Can you work these out from the model? Positions are in its coordinate system, mm. A direction names the side the tool comes from. Coordinates: 2 decimals unless noted, no trailing zeros. Order: outer loops, then holes, each group sorted by start corner. A loop starts at its lowest first (then second) coordinate and runs counter-clockwise, first axis right, second up. Notation, with made-up numbers: (17, -28.5) -> (43, -28.5) arc R22 cw to (43, 5.5) -> close; hole circle Ø9 at (26, 33.25). An arc over 180 degrees is marked (long way). Write item = value, one per line. Start each with the question number.
from build123d import *

# Parameters (mm, degrees)
SKETCH1_W               = 60
SKETCH1_H               = 60
BOSS_EXTRUDE1_DEPTH     = 85
SKETCH2_W               = 40
SKETCH2_H               = 35
CUT_EXTRUDE1_DEPTH      = 121.104121495
CUT_EXTRUDE2_DEPTH      = 99.488578018
CUT_EXTRUDE2_DEPTH_BACK = 99.488578018
SKETCH3_R               = 11


with BuildPart() as part:
    # Sketch1 → Boss-Extrude1 (new body)
    with BuildSketch(Plane(origin=(0, 0, 0), x_dir=(1, 0, 0), z_dir=(0, 1, 0))):
        with Locations((30, 30)):
            Rectangle(SKETCH1_W, SKETCH1_H)
    extrude(amount=BOSS_EXTRUDE1_DEPTH)

    # Sketch2 → Cut-Extrude1 (cut, through all)
    with BuildSketch(Plane(origin=(60, 0, 0), x_dir=(0, 0, -1), z_dir=(1, 0, 0))):
        with Locations((20, 52.5)):
            Rectangle(SKETCH2_W, SKETCH2_H)
    extrude(amount=-CUT_EXTRUDE1_DEPTH, mode=Mode.SUBTRACT)

    # Sketch3 → Cut-Extrude2 (cut, two sides: drawn at the far end of the back side and taken through both)
    with BuildSketch(Plane(origin=(0, 35, 0), x_dir=(1, 0, 0), z_dir=(0, 1, 0)).offset(-CUT_EXTRUDE2_DEPTH_BACK)):
        with Locations(Location((30, 20, 0), (0, 0, 270))):
            Circle(SKETCH3_R)
    extrude(amount=CUT_EXTRUDE2_DEPTH + CUT_EXTRUDE2_DEPTH_BACK, mode=Mode.SUBTRACT)


solid = part.part
(1) Imagine slicing it at B-B (z = -4.5). Write out the boundary of the cut face in (x, y), plus the area to 3 significant figures.
(2) If I drill on L1, parallel to Z at x = 30, y = 22; L2, parallel to Y at x = 30, z = -6; L3, parallel to X at y = 73, z = -20, over which ranges is the centre line in solid material (lowest first)? Write a range as from..to.
(3) Imagine slicing it at C-C (z = -20). Write out the boundary of the cut face in (x, y).
(4) For P1, Ø2, axis at x = 52.5, y = 41.5, coming from the +Z side, with a flat end and sliding along its axis, tell me the tip position at first contact or that it passes through.
(5) Imagine slicing it at D-D (x = 46.5). Write out the boundary of the cut face in (y, z), plus the area to 3 significant figures.
(6) For faces 1 (the face through (30, 77, 0)), 2 (the face through (37, 35, -11)), which set-ups out of +Z, -Z, +X, -X, +Y, -Y let a thin tool reach every point of the face, with its end or its side?
(7) Imagine slicing it at A-A (x = 30). Write out the boundary of the cut face in (y, z), plus the area to 3 significant figures.
(8) Thinking about a two-plate mould opening in X: for faces 3 (the face through (25.787, 77.395, -9.839)), 4 (the face through (60, 32, -30)), 5 (the face through (30, 85, -37)), which applies, +X half, -X half, draft (parallel to the pull), parting line (faces both ways), or undercut?
Result set:
q1.outline = (0, 0) -> (60, 0) -> (60, 35) -> (0, 35) -> close; (0, 70) -> (60, 70) -> (60, 85) -> (0, 85) -> close
q1.area = 3,000 mm2
q2.L1 = -60..-31, -9..0
q2.L2 = 0..35, 70..85
q2.L3 = 0..19, 41..60
q3.outline = (0, 0) -> (19, 0) -> (19, 35) -> (0, 35) -> close; (0, 70) -> (19, 70) -> (19, 85) -> (0, 85) -> close; (41, 0) -> (60, 0) -> (60, 35) -> (41, 35) -> close; (41, 70) -> (60, 70) -> (60, 85) -> (41, 85) -> close
q4.P1 = -40
q5.outline = (0, -60) -> (85, -60) -> (85, 0) -> (70, 0) -> (70, -40) -> (35, -40) -> (35, 0) -> (0, 0) -> close
q5.area = 3,700 mm2
q6.face_1 = +Z, +X, -X, +Y, -Y
q6.face_2 = +Z, +X, -X
q7.outline = (0, -60) -> (85, -60) -> (85, -31) -> (70, -31) -> (70, -40) -> (35, -40) -> (35, -31) -> (0, -31) -> close; (0, -9) -> (35, -9) -> (35, 0) -> (0, 0) -> close; (70, -9) -> (85, -9) -> (85, 0) -> (70, 0) -> close
q7.area = 2,600 mm2
q8.face_3 = undercut
q8.face_4 = +X half
q8.face_5 = draft
